CAD build for the part. Positions are in the model's coordinates, mm. Face numbers are marked on the shaded views. Coordinates: 2 decimals unless noted, no trailing zeros. Loops run counter-clockwise (first coordinate to the right, second up) from the corner with the lowest first, then second, coordinate; pieces in that order, holes last. Notation, with made-up numbers: (63, 61) -> (80, 61) arc R16 ccw to (80, 78) -> close; hole circle Ø11 at (85.25, -33). An arc over 180 degrees is marked (long way). Answer as CSV lines item,"result". Start each with the question number.
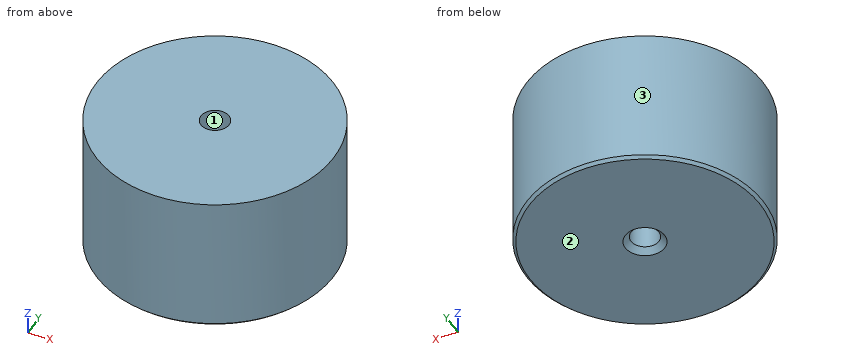
```python
from build123d import *

# Parameters (mm, degrees)
F0_R     = 21
F0_R_2   = 2.5
F1_DEPTH = 25
F2_SIZE  = 1
F3_SIZE  = 0.5


with BuildPart() as f1:
    # F0 (on Top) → F1 (new body)
    with BuildSketch(Plane.XY):
        Circle(F0_R)
        Circle(F0_R_2, mode=Mode.SUBTRACT)
    extrude(amount=F1_DEPTH)

    # F2
    f2_edges = [f1.edges().sort_by_distance(p)[0] for p in [
        (-2.5, 0, 0),
    ]]
    chamfer(f2_edges, length=F2_SIZE)

    # F3
    f3_edges = [f1.edges().sort_by_distance(p)[0] for p in [
        (-21, 0, 0),
    ]]
    chamfer(f3_edges, length=F3_SIZE)


solid = f1.part
```
Q1. Two-plate mould, pull along X, no slides. Class the marked faces 1, 2 and 3: pulls with the +X half, pulls with the -X half, needs draft (parallel to the pull), parting line crosses it, or undercut.
Q2. Saw through at C-C (z = 5.75). List the corners of the cut face in (x, y), and give its area (3 significant figures).
Q3. Probe probe 1 along Y at (x, z) = (0, 13.25); probe 2 along X at (y, z) = (3, 7.5); probe 3 along X at (y, z) = (7, 16.5). List the from-to ranges inside material, lowest first. Write a range as from..to.
Q4. Saw through at A-A (y = 0). List the corners of the cut face in (x, z), and give its area (3 significant figures).
Q5. Pin check, flat tips, straight feed: pin 1 Ø5 at (x, z) = (-13, 5.5) entering from +Y; pin 2 Ø10 at (x, z) = (-6, 18.5) entering from +Y; pin 3 Ø3 at (x, z) = (-5.5, 5) entering from -Y. Stop position of each tip, or through.
Ans:
1,face 1,"undercut"
1,face 2,"needs draft"
1,face 3,"parting line crosses it"
2,outline,"circle Ø42 at (0, 0); hole circle Ø5 at (0, 0)"
2,area,"1,370 mm²"
3,probe 1,"y = -21..-2.5, 2.5..21"
3,probe 2,"x = -20.78..20.78"
3,probe 3,"x = -19.8..19.8"
4,outline,"(-21, 0.5) -> (-20.5, 0) -> (-3.5, 0) -> (-2.5, 1) -> (-2.5, 25) -> (-21, 25) -> close; (2.5, 1) -> (3.5, 0) -> (20.5, 0) -> (21, 0.5) -> (21, 25) -> (2.5, 25) -> close"
4,area,"924 mm²"
5,pin 1,"stops at y = 18.19"
5,pin 2,"stops at y = 20.98"
5,pin 3,"stops at y = -20.62"
